Source: CAD feature listing. Evaluate the final solid. Frame: model axes, mm. Round coordinates to 2 decimals unless told otherwise and drop trailing zeros. Loops run counter-clockwise (first coordinate to the right, second up) from the corner with the lowest first, then second, coordinate; pieces in that order, holes last. Notation, with made-up numbers: M -4,-9.75 L 48,-9.75 A24 ccw 48,26.25 Z; hole C 16.5,21 d3. An arc over 180 degrees is marked long. Write each question's results on one line, items separated by ' | '. Start each with the question number.
1. Ray query, line 1 (Z direction, x = 207.5, y = 17); line 2 (Z direction, x = 56.5, y = 6.25); line 3 (Z direction, x = 210.5, y = 7). Return the intervals inside material, ascending.
2. Section C-C on z = -127.5. Output: boundary loops of the cut face in (x, y).
3. Section A-A on y = 10.5. Give the number of separate pieces and of enclosed holes in the cut face, and give its area (3 significant figures).
4. Contact query for flat-ended pins moving along their axis: pin 1 Ø6 at (x, z) = (210.02, 10.02) entering from -Y; pin 2 Ø6 at (x, y) = (86.5, 12) entering from -Z; pin 3 Ø5 at (x, y) = (158.5, 3.5) entering from +Z; pin 4 Ø3 at (y, z) = (6.5, -172) entering from -X. Output: stop coordinate, or through.
5. Section B-B on x = 110.5. Output: boundary loops of the cut face in (y, z).
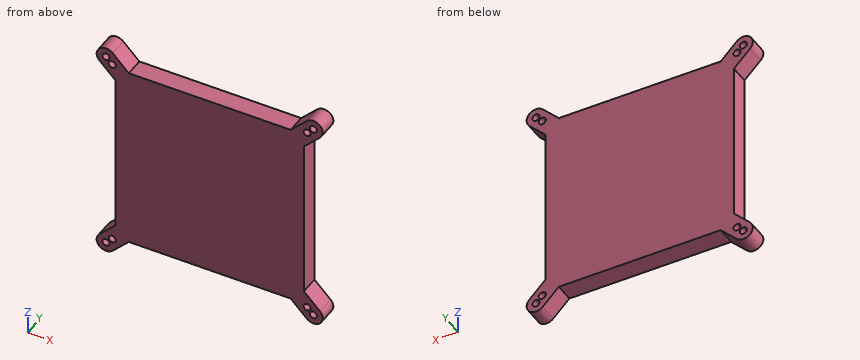
from build123d import *

# Parameters (mm, degrees)
SKETCH1_W               = 200
SKETCH1_H               = 200
BOSS_EXTRUDE1_DEPTH     = 20
SKETCH2_R               = 3.7970867
BOSS_EXTRUDE2_DEPTH     = 20
MIRROR4_COPY_1_SKETCH_R = 3.7970867
MIRROR4_COPY_1_DEPTH    = 20


with BuildPart() as part:
    # Sketch1 → Boss-Extrude1 (new body)
    with BuildSketch(Plane(origin=(0, 0, 0), x_dir=(1, 0, 0), z_dir=(0, 1, 0))):
        with Locations((100, 100)):
            Rectangle(SKETCH1_W, SKETCH1_H)
    extrude(amount=BOSS_EXTRUDE1_DEPTH)

    # Sketch2 → Boss-Extrude2 (add)
    with BuildSketch(Plane.XZ):
        with BuildLine():
            Line((0, -14.142135624), (-17.087625271, 2.945489647))
            ThreePointArc((-17.087625271, 2.945489647), (-17.087625271, 17.087625271), (-2.945489647, 17.087625271))
            Line((-2.945489647, 17.087625271), (14.142135624, 0))
            Line((14.142135624, 0), (0, 0))
            Line((0, 0), (0, -14.142135624))
        make_face()
        with Locations((-10.016557459, 10.016557459)):
            Circle(SKETCH2_R, mode=Mode.SUBTRACT)
        with Locations((-3.415367361, 3.415367361)):
            Circle(SKETCH2_R, mode=Mode.SUBTRACT)
    boss_extrude2 = extrude(amount=-BOSS_EXTRUDE2_DEPTH)

    # Mirror3: Boss-Extrude2 across plane
    add(boss_extrude2.mirror(Plane(origin=(100, 0, 0), x_dir=(0, 0, 1), z_dir=(1, 0, 0))))

    # Mirror4: Boss-Extrude2 across plane
    add(boss_extrude2.mirror(Plane(origin=(0, 0, -100), x_dir=(1, 0, 0), z_dir=(0, 0, -1))))

    # Mirror4 copy 1 sketch → Mirror4 copy 1 (add)
    with BuildSketch(Plane(origin=(200, 0, -200), x_dir=(-1, 0, 0), z_dir=(0, -1, 0))):
        with BuildLine():
            Line((0, -14.142135624), (-17.087625271, 2.945489647))
            ThreePointArc((-17.087625271, 2.945489647), (-17.087625271, 17.087625271), (-2.945489647, 17.087625271))
            Line((-2.945489647, 17.087625271), (14.142135624, 0))
            Line((14.142135624, 0), (0, 0))
            Line((0, 0), (0, -14.142135624))
        make_face()
        with Locations((-10.016557459, 10.016557459)):
            Circle(MIRROR4_COPY_1_SKETCH_R, mode=Mode.SUBTRACT)
        with Locations((-3.415367361, 3.415367361)):
            Circle(MIRROR4_COPY_1_SKETCH_R, mode=Mode.SUBTRACT)
    extrude(amount=-MIRROR4_COPY_1_DEPTH)


solid = part.part
Taken from the geometry:
1) line 1: -219.69 to -212.86, -207.17 to -193.36, -6.64 to 7.17, 12.86 to 19.69 | line 2: -200 to 0 | line 3: -220 to -213.78, -206.25 to -196.36, -3.64 to 6.25, 13.78 to 20
2) outline: M 0,0 L 200,0 L 200,20 L 0,20 Z
3) separate pieces: 1 | enclosed holes: 8 | area: 41,800 mm^2
4) pin 1: through | pin 2: z = -200 | pin 3: z = 0 | pin 4: x = 0
5) outline: M 0,-200 L 20,-200 L 20,0 L 0,0 Z
